Read the model definition and answer for the solid it produces. Units are mm, in the model's axes. A direction names the side the tool comes from. Coordinates: 2 decimals unless noted, no trailing zeros. Order: outer loops, then holes, each group sorted by start corner. A loop starts at its lowest first (then second) coordinate and runs counter-clockwise, first axis right, second up. Notation, with made-up numbers: (42.25, 30.25) -> (77.25, 30.25) arc R29 cw to (77.25, 66.25) -> close; hole circle Ø1 at (70.5, -35.75). An arc over 180 degrees is marked (long way). Use CSV: the item, a comma, the result in double quotes.
```python
from build123d import *

# Parameters (mm, degrees)
SKETCH1_W                        = 5.5
SKETCH1_H                        = 11
MAIN_BASE_DEPTH                  = 101.61
SIDE_CUT_OUT_DEPTH               = 89.61
TOP_RUBBER_BAND_CUT_OUT_DEPTH    = 103.351561297
BOTTOM_RUBBER_BAND_CUT_OUT_DEPTH = 103.351561297
SKETCH6_W                        = 1.75
SKETCH6_H                        = 11
MOTOR_PULLEY_CUT_OUT_DEPTH       = 12
SKETCH7_W                        = 1.75
SKETCH7_H                        = 11
PULLEY_CUT_OUT_DEPTH             = 10
SKETCH11_R                       = 1.5
MOTOR_SHAFT_CUT_OUT_DEPTH        = 103.272452792
SNAP_START                       = 5.27
SNAP_HOOK_DRIVEN_SIDE_DEPTH      = 0.23
SNAP_START_2                     = -97.613689555
SNAP_HOOK_DRIVEN_SIDE_2_DEPTH    = 4.266231519
SNAP_START_3                     = -97.666097334
SNAP_HOOK_DRIVEN_SIDE_3_DEPTH    = 4.371047077
SNAP_START_4                     = 3
SNAP_HOOK_DRIVEN_SIDE_4_DEPTH    = 4
SKETCH16_W                       = 2
SKETCH16_H                       = 6
SNAP_HOOK_BASE_DEPTH             = 12
SNAP_HOOK_BASE_CHAMFER_SIZE      = 2
SNAP_HOOK_GUIDE_SIDE_DEPTH       = 0.23
SNAP_START_5                     = -8.132595504
SNAP_HOOK_GUIDE_SIDE_2_DEPTH     = 4.266231519
SNAP_START_6                     = -8.185003283
SNAP_HOOK_GUIDE_SIDE_3_DEPTH     = 4.371047078
SNAP_HOOK_GUIDE_SIDE_4_DEPTH     = 4
SKETCH13_W                       = 1
SKETCH13_H                       = 0.5
BOSS_EXTRUDE3_DEPTH              = 12
RAIL_CHAMFER_SIZE                = 0.5


with BuildPart() as part:
    # Sketch1 → main_base (new body)
    with BuildSketch(Plane.XY):
        with Locations((2.75, 5.5)):
            Rectangle(SKETCH1_W, SKETCH1_H)
    extrude(amount=-MAIN_BASE_DEPTH)

    # Sketch3 → side_cut_out (cut)
    with BuildSketch(Plane.XY):
        Polygon((5.5, 9), (3.5, 7), (3.5, 0), (5.5, 0), align=None)
    extrude(amount=-SIDE_CUT_OUT_DEPTH, mode=Mode.SUBTRACT)

    # Sketch4 → top_rubber_band_cut_out (cut, through all)
    with BuildSketch(Plane.XY):
        Polygon((0, 7.3), (0, 11), (2.7, 11), (2.7, 10), align=None)
    extrude(amount=-TOP_RUBBER_BAND_CUT_OUT_DEPTH, mode=Mode.SUBTRACT)

    # Sketch5 → bottom_rubber_band_cut_out (cut, through all)
    with BuildSketch(Plane.XY):
        Polygon((2, 0), (0, 2), (0, 0), align=None)
    extrude(amount=-BOTTOM_RUBBER_BAND_CUT_OUT_DEPTH, mode=Mode.SUBTRACT)

    # Sketch6 → motor_pulley_cut_out (cut)
    with BuildSketch(Plane(origin=(0, 0, -101.61), x_dir=(-1, 0, 0), z_dir=(0, 0, -1))):
        with Locations((-0.875, 5.5)):
            Rectangle(SKETCH6_W, SKETCH6_H)
    extrude(amount=-MOTOR_PULLEY_CUT_OUT_DEPTH, mode=Mode.SUBTRACT)

    # Sketch7 → pulley_cut_out (cut)
    with BuildSketch(Plane.XY):
        with Locations((0.875, 5.5)):
            Rectangle(SKETCH7_W, SKETCH7_H)
    extrude(amount=-PULLEY_CUT_OUT_DEPTH, mode=Mode.SUBTRACT)

    # Sketch10 → half_circle_cut_out (revolve, cut)
    with BuildSketch(Plane(origin=(0, 5, 0), x_dir=(1, 0, 0), z_dir=(0, 1, 0))):
        with BuildLine():
            Line((1.5, 5), (1.5, 3.75))
            ThreePointArc((1.5, 3.75), (2.383883476, 4.116116524), (2.75, 5))
            Line((2.75, 5), (1.5, 5))
        make_face()
    revolve(axis=Axis((2.75, 5, -5), (-1, 0, 0)), mode=Mode.SUBTRACT)

    # Sketch11 → motor_shaft_cut_out (cut, through all)
    with BuildSketch(Plane.ZY.offset(-1.75)):
        with Locations((-95.61, 5)):
            Circle(SKETCH11_R)
    extrude(amount=-MOTOR_SHAFT_CUT_OUT_DEPTH, mode=Mode.SUBTRACT)



with BuildPart() as body_2:
    # Snap Hook Driven Side: read off the stored shape, not the designer's step
    # Snap Hook Driven Side outline → Snap Hook Driven Side (new body)
    with BuildSketch(Plane.YZ.offset(SNAP_START)):
        Polygon((-1, -97.613689555), (-1, -93.347458036), (-3.54, -93.480573796), (-3.54, -97.480573796), align=None)
    extrude(amount=SNAP_HOOK_DRIVEN_SIDE_DEPTH)


with BuildPart() as part_1:
    add(part.part)

    add(body_2.part)  # Snap Hook Driven Side 2 merges body 2
    # Snap Hook Driven Side 2 outline → Snap Hook Driven Side 2 (add)
    with BuildSketch(Plane.XY.offset(SNAP_START_2)):
        Polygon((5.5, 0), (3.5, 0), (5.27, -3.54), (5.27, -1), (5.5, -1), align=None)
        Polygon((6.5, -1), (5.5, -1), (5.5, -3.54), align=None)
    extrude(amount=SNAP_HOOK_DRIVEN_SIDE_2_DEPTH)

    # Snap Hook Driven Side 3 outline → Snap Hook Driven Side 3 (add)
    with BuildSketch(Plane.XY.offset(SNAP_START_3)):
        Polygon((5.5, 0), (3.5, 0), (5.27, -3.54), (5.27, -1), (5.5, -1), align=None)
    extrude(amount=SNAP_HOOK_DRIVEN_SIDE_3_DEPTH)

    # Snap Hook Driven Side 4 outline → Snap Hook Driven Side 4 (cut)
    with BuildSketch(Plane.YZ.offset(SNAP_START_4)):
        Polygon((0, -93.295050257), (-5, -93.295050257), (-5, -93.557089154), (-3.54, -93.480573796), align=None)
        Polygon((-3.54, -97.480573796), (-5, -97.404058439), (-5, -97.666097334), (0, -97.666097334), align=None)
    extrude(amount=SNAP_HOOK_DRIVEN_SIDE_4_DEPTH, mode=Mode.SUBTRACT)

    # Sketch16 → Snap Hook Base (add)
    with BuildSketch(Plane.XY):
        with Locations((4.5, 3)):
            Rectangle(SKETCH16_W, SKETCH16_H)
    extrude(amount=-SNAP_HOOK_BASE_DEPTH)

    # Snap Hook Base Chamfer
    snap_hook_base_chamfer_edges = [part_1.edges().sort_by_distance(p)[0] for p in [
        (5.5, 6, -6),
    ]]
    chamfer(snap_hook_base_chamfer_edges, length=SNAP_HOOK_BASE_CHAMFER_SIZE - 0.0001)  # a hair under: the kernel refuses the full size



with BuildPart() as body_2_2:
    # Snap Hook Guide Side: read off the stored shape, not the designer's step
    # Snap Hook Guide Side outline → Snap Hook Guide Side (new body)
    with BuildSketch(Plane.YZ.offset(SNAP_START)):
        Polygon((-1, -3.866363984), (-3.54, -3.999479744), (-3.54, -7.999479744), (-1, -8.132595504), align=None)
    extrude(amount=SNAP_HOOK_GUIDE_SIDE_DEPTH)


with BuildPart() as part_2:
    add(part_1.part)

    add(body_2_2.part)  # Snap Hook Guide Side 2 merges body 2 2
    # Snap Hook Guide Side 2 outline → Snap Hook Guide Side 2 (add)
    with BuildSketch(Plane.XY.offset(SNAP_START_5)):
        Polygon((5.27, -1), (5.5, -1), (5.5, 0), (3.5, 0), (5.27, -3.54), align=None)
        Polygon((6.5, -1), (5.5, -1), (5.5, -3.54), align=None)
    extrude(amount=SNAP_HOOK_GUIDE_SIDE_2_DEPTH)

    # Snap Hook Guide Side 3 outline → Snap Hook Guide Side 3 (add)
    with BuildSketch(Plane.XY.offset(SNAP_START_6)):
        Polygon((5.27, -1), (5.5, -1), (5.5, 0), (3.5, 0), (5.27, -3.54), align=None)
    extrude(amount=SNAP_HOOK_GUIDE_SIDE_3_DEPTH)

    # Snap Hook Guide Side 4 outline → Snap Hook Guide Side 4 (cut)
    with BuildSketch(Plane.YZ.offset(SNAP_START_4)):
        Polygon((0, -3.813956205), (-5, -3.813956205), (-5, -4.075995102), (-3.54, -3.999479744), align=None)
        Polygon((-3.54, -7.999479744), (-5, -7.922964386), (-5, -8.185003283), (0, -8.185003283), align=None)
    extrude(amount=SNAP_HOOK_GUIDE_SIDE_4_DEPTH, mode=Mode.SUBTRACT)

    # final_mirror: part across plane


with BuildPart() as part_3:
    add(part_2.part)
    add(part_2.part.mirror(Plane(origin=(0, 0, 0), x_dir=(0, 0, 1), z_dir=(1, 0, 0))))

    # Sketch13 → Boss-Extrude3 (add)
    with BuildSketch(Plane(origin=(0, 0, -101.61), x_dir=(-1, 0, 0), z_dir=(0, 0, -1))):
        Polygon((7.25, 11), (5.5, 11), (5.5, 10), (6.25, 10), (7.25, 10), align=None)
        with Locations((6.75, 9.75)):
            Rectangle(SKETCH13_W, SKETCH13_H)
    extrude(amount=-BOSS_EXTRUDE3_DEPTH)

    # rail_chamfer
    rail_chamfer_edges = [part_3.edges().sort_by_distance(p)[0] for p in [
        (-5.5, 11, -44.805),
        (-7.25, 11, -95.61),
        (5.5, 11, -50.805),
    ]]
    chamfer(rail_chamfer_edges, length=RAIL_CHAMFER_SIZE)


solid = part_3.part
```
Item 1: The mould has two halves that part along X. Classify faces 1 (the flat face through (4.5, 5, -5.9)), 2 (the flat face through (-4.5, 8, -44.2)), 3 (the flat face through (0, 5, -10)): +X half, -X half, draft (parallel to the pull), parting line (faces both ways), or undercut.
Return value:
face 1,"+X half"
face 2,"-X half"
face 3,"undercut"
Item 2: Find section B-B, the plane y = 5. Give the number of separate pieces and of enclosed holes in the cut face, then the cut area to 3 significant figures.
Return value:
separate pieces,"3"
enclosed holes,"0"
area,"680 mm^2"
Item 3: Each of these flat-tipped pins is pushed along its axis until it touches: P1, Ø6, axis at x = -3.5, z = -20.5, coming from the -Y side; P2, Ø1, axis at y = 9, z = -76, coming from the -X side; P3, Ø4, axis at y = 2, z = -59, coming from the -X side. Where does it stop, or does it pass through?
Return value:
P1,"stops at y = 0"
P2,"stops at x = -5.5"
P3,"stops at x = -3.5"
Item 4: Find section A-A, the plane z = -65. Give the vertices of the cut face in (x, y), then the cut area to 3 significant figures.
Return value:
outline,"(-5.5, 9) -> (-3.5, 7) -> (-3.5, 0) -> (-2, 0) -> (0, 2) -> (2, 0) -> (3.5, 0) -> (3.5, 7) -> (5.5, 9) -> (5.5, 10.5) -> (5, 11) -> (2.7, 11) -> (2.7, 10) -> (0, 7.3) -> (-2.7, 10) -> (-2.7, 11) -> (-5, 11) -> (-5.5, 10.5) -> close"
area,"72.1 mm^2"
Item 5: A tool of negligible diameter and unlimited length cuts with its end or side. For faces 4 (the flat face through (4, 2, -12)), 5 (the flat face through (-5.5, 2, -6)), 6 (the flat face through (1.75, 3.6, -4.9)), from which of +Z, -Z, +X, -X, +Y, -Y can it reach the whole face along a straight path? Write none if from no direction.
Return value:
face 4,"+X, -Y"
face 5,"+Z, -Z, -X, +Y"
face 6,"+Z, +Y, -Y"
Item 6: Straight lines are drawn through the part: line 1 along X through (y, z) = (6.75, -92); line 2 along X through (y, z) = (4.25, -42.5); line 3 along X through (y, z) = (8, -54). For each, find the intervals that lie inside material, in ascending order.
Return value:
line 1,"x = -5.5 to -1.75, 1.75 to 5.5"
line 2,"x = -3.5 to 3.5"
line 3,"x = -4.5 to -0.7, 0.7 to 4.5"
